Autodesk Inventor part; units mm, degrees
ref_plane "YZ Plane" through (0, 0, 0) normal (1, 0, 0) x (0, 1, 0)
ref_plane "XZ Plane" through (0, 0, 0) normal (0, 1, 0) x (-1, 0, 0)
ref_plane "XY Plane" through (0, 0, 0) normal (0, 0, 1) x (1, 0, 0)
sketch "Szkic1" plane through (0, 0, 0) normal (0, 1, 0) x (-1, 0, 0)
  line L0 (-59.65, -33) -> (59.65, -33)
  line L1 (59.65, -33) -> (59.65, 33)
  line L2 (59.65, 33) -> (-59.65, 33)
  line L3 (-59.65, 33) -> (-59.65, -33)
  line L4 (-59.65, -33) -> (59.65, 33) construction
  line L5 (59.65, -33) -> (-59.65, 33) construction
  point P0 (0, 0)
  dimension "d0" = 119.3
  dimension "d1" = 66
extrude "Wyciągnięcie proste1" add sketch "Szkic1" along normal blind 1.5
sketch "Szkic3" plane through (0, 1.5, 0) normal (0, 1, 0) x (1, 0, 0)
  line L0 (54.15, -28) -> (-24.59, -28)
  line L1 (-24.59, -28) -> (-24.59, -23)
  line L2 (-24.59, -23) -> (54.15, -23)
  line L3 (54.15, -23) -> (54.15, -28)
  line L4 (-59.65, -33) -> (59.65, -33)
  line L5 (59.65, -33) -> (59.65, 33)
  line L6 (83.51, 0) -> (-83.51, 0)
  point P0 (0, 0)
  dimension "d9" = 78.74
  dimension "d10" = 5
  dimension "d11" = 5
  dimension "d12" = 5.5
extrude "Wyciągnięcie proste6" add sketch "Szkic3" along normal blind 5
sketch "Szkic4" plane through (0, 1.5, 0) normal (0, 1, 0) x (1, 0, 0)
  line L0 (-34.15, -25.5) -> (-49.65, -25.5)
  line L1 (-49.65, -25.5) -> (-49.65, -28)
  line L2 (-49.65, -28) -> (-34.15, -28)
  line L3 (-34.15, -28) -> (-34.15, -25.5)
  line L4 (-59.65, -33) -> (59.65, -33)
  line L5 (-59.65, 33) -> (-59.65, -33)
  point P0 (0, 0)
  dimension "d17" = 15.5
  dimension "d18" = 2.5
  dimension "d61" = 10
  dimension "d62" = 5
extrude "Wyciągnięcie proste4" add sketch "Szkic4" along normal blind 8.5
sketch "Szkic5" plane through (0, 1.5, 0) normal (0, 1, 0) x (1, 0, 0)
  line L0 (53.65, 21) -> (-6.35, 21)
  line L1 (-6.35, 21) -> (-6.35, -21.5)
  line L2 (-6.35, -21.5) -> (53.65, -21.5)
  line L3 (53.65, -21.5) -> (53.65, 21)
  line L4 (53.65, 21) -> (-6.35, -21.5) construction
  line L5 (-6.35, 21) -> (53.65, -21.5) construction
  line L6 (59.65, -33) -> (59.65, 33)
  line L7 (-59.65, -33) -> (59.65, -33)
  point P0 (0, 0)
  point P1 (23.65, -0.25)
  dimension "d25" = 60
  dimension "d26" = 42.5
  dimension "d28" = 6
  dimension "d36" = 11.5
extrude "Wyciągnięcie proste5" add sketch "Szkic5" along normal blind 5
pattern_linear "Szyk prostokątny1" count 2 spacing 50.5 along (0, 0, -1) of "Wyciągnięcie proste6"
sketch "Szkic6" plane through (0, 1.5, 0) normal (0, 1, 0) x (1, 0, 0)
  line L0 (-51.15, -4) -> (-61.15, -4)
  line L1 (-61.15, -4) -> (-61.15, 5)
  line L2 (-61.15, 5) -> (-51.15, 5)
  line L3 (-51.15, 5) -> (-51.15, -4)
  line L4 (-51.15, -4) -> (-61.15, 5) construction
  line L5 (-61.15, -4) -> (-51.15, 5) construction
  line L6 (-59.65, -33) -> (59.65, -33)
  line L7 (-59.65, 33) -> (-59.65, -33)
  point P0 (0, 0)
  point P1 (-56.15, 0.5)
  dimension "d37" = 10
  dimension "d38" = 9
  dimension "d39" = 29
  dimension "d40" = 1.5
extrude "Wyciągnięcie proste7" add sketch "Szkic6" along normal blind 5
sketch "Szkic7" plane through (0, 1.5, 0) normal (0, 1, 0) x (1, 0, 0)
  circle A0 centre (-23.65, -13) radius 2.75
  line L0 (-59.65, 33) -> (-59.65, 5)
  circle A1 centre (-23.65, 12.5) radius 2.75
  line L1 (-59.65, -33) -> (59.65, -33)
  point P0 (0, 0)
  dimension "d43" = 5.5
  dimension "d46" = 25.5
  dimension "d51" = 20
  dimension "d52" = 36
extrude "Wyciągnięcie proste8" add sketch "Szkic7" along normal blind 10.5
sketch "Szkic8" plane through (0, 1.5, 0) normal (0, 1, 0) x (1, 0, 0)
  line L0 (-32.65, -17.5) -> (-48.15, -17.5)
  line L1 (-48.15, -17.5) -> (-48.15, 27)
  line L2 (-48.15, 27) -> (-32.65, 27)
  line L3 (-32.65, 27) -> (-32.65, -17.5)
  line L4 (-32.65, -17.5) -> (-48.15, 27) construction
  line L5 (-48.15, -17.5) -> (-32.65, 27) construction
  line L6 (-59.65, -33) -> (59.65, -33)
  line L7 (-59.65, -4) -> (-59.65, -33)
  point P0 (0, 0)
  point P1 (-40.4, 4.75)
  dimension "d55" = 15.5
  dimension "d56" = 27
  dimension "d57" = 44.5
  dimension "d58" = 15.5
extrude "Wyciągnięcie proste9" add sketch "Szkic8" along normal blind 8
properties part number "stm32f429"
Design review of the part built by this model. Coordinates are the model's own, in mm. A direction names the side the tool comes from. Round coordinates to 2 decimals unless told otherwise and drop trailing zeros. Loops run counter-clockwise (first coordinate to the right, second up) from the corner with the lowest first, then second, coordinate; pieces in that order, holes last. Notation, with made-up numbers: (45, 69) - (78, 69) arc R25 ccw to (78, 87) - close; hole circle Ø1 at (74, 12.25). An arc over 180 degrees is marked (long way). One line per question, with ' | ' between items.
1. We need section D-D, the plane z = -18.5. State the section outline as (x, y) points, and give its area (3 significant figures).
Results are:
outline: (-59.65, 0) - (59.65, 0) - (59.65, 1.5) - (53.65, 1.5) - (53.65, 6.5) - (-6.35, 6.5) - (-6.35, 1.5) - (-32.65, 1.5) - (-32.65, 9.5) - (-48.15, 9.5) - (-48.15, 1.5) - (-59.65, 1.5) - close | area: 603 mm²
2. Draft analysis for pull direction Z (two halves, no side actions). For faces 1 (the face through (-41, 5, -27)), 2 (the face through (14, 6.5, -25)), 3 (the face through (-21.03, 6.68, -11.67)), state which applies: released by +Z, released by -Z, zero draft, split by the parting line, or undercut.
Results are:
face 1: released by -Z | face 2: zero draft | face 3: undercut
3. We need section A-A, the plane y = 8. State the section outline as (x, z) points.
Results are:
outline: (-49.65, 25.5) - (-34.15, 25.5) - (-34.15, 28) - (-49.65, 28) - close; (-48.15, -27) - (-32.65, -27) - (-32.65, 17.5) - (-48.15, 17.5) - close; circle Ø5.5 at (-23.65, -12.5); circle Ø5.5 at (-23.65, 13)
4. We need section C-C, the plane z = 13. State the section outline as (x, y) points, and give its area (3 significant figures).
Results are:
outline: (-59.65, 0) - (59.65, 0) - (59.65, 1.5) - (53.65, 1.5) - (53.65, 6.5) - (-6.35, 6.5) - (-6.35, 1.5) - (-20.9, 1.5) - (-20.9, 12) - (-26.4, 12) - (-26.4, 1.5) - (-32.65, 1.5) - (-32.65, 9.5) - (-48.15, 9.5) - (-48.15, 1.5) - (-59.65, 1.5) - close | area: 661 mm²
5. For faces 4 (the face through (-56, 4, 4)), 5 (the face through (15, 4, 28)), 6 (the face through (-41, 9.5, -5)), list the 3-axis set-ups (+Z, -Z, +X, -X, +Y, -Y) from which the entire face can be reached by the end or side of a thin tool; tool diameter is ignored.
Results are:
face 4: +Z, -X, +Y | face 5: +Z, +X, -X, +Y | face 6: -Z, -X, +Y
6. Clearance check with flat-ended pins moving along their axes: P1, Ø1.5, axis at y = 4, z = 10.5, coming from the -X side; P2, Ø2, axis at x = 35.5, z = 14, coming from the +Y side; P3, Ø5.5, axis at x = 16.5, y = 5, coming from the +Z side. State where each tip first meets the part, or that it passes through.
Results are:
P1: stops at x = -48.15 | P2: stops at y = 6.5 | P3: stops at z = 28
7. We need section B-B, the plane x = -54. State the section outline as (y, z) points, and give its area (3 significant figures).
Results are:
outline: (0, -33) - (1.5, -33) - (1.5, -5) - (6.5, -5) - (6.5, 4) - (1.5, 4) - (1.5, 33) - (0, 33) - close | area: 144 mm²
8. For L1, parallel to X at y = 5, z = -3.5; L2, parallel to Z at x = -8.5, y = 6.25; L3, parallel to X at y = 6, z = 26, list the stretches that pass through material, from the lowest coordinate up. Write a range as [from, to].
Results are:
L1: x = [-61.15, -51.15], [-48.15, -32.65], [-6.35, 53.65] | L2: z = [-27.5, -22.5], [23, 28] | L3: x = [-49.65, -34.15], [-24.59, 54.15]
